Autodesk Inventor part; units mm, degrees
ref_plane "YZ Plane" through (0, 0, 0) normal (1, 0, 0) x (0, 1, 0)
ref_plane "XZ Plane" through (0, 0, 0) normal (0, 1, 0) x (-1, 0, 0)
ref_plane "XY Plane" through (0, 0, 0) normal (0, 0, 1) x (1, 0, 0)
sketch "Sketch1" plane through (0, 0, 0) normal (0, 1, 0) x (-1, 0, 0)
  line L0 (0, 0) -> (-60.96, 0)
  line L1 (-60.96, 0) -> (-60.96, -111.76)
  line L2 (-60.96, -111.76) -> (0, -111.76)
  line L3 (0, -111.76) -> (0, 0)
  dimension "d0" = 60.96
  dimension "d1" = 111.76
extrude "Extrusion1" add sketch "Sketch1" along normal blind 31.75 draft -2
fillet "Fillet1" radius 6.35 4 edges at (60.4056, 15.875, -0.5544) (60.4056, 15.875, -111.2056) (0.5544, 15.875, -111.2056) (0.5544, 15.875, -0.5544)
fillet "Fillet2" radius 0.635 16 edges at (57.993, 31.75, -2.967) (30.48, 31.75, -1.1087) (2.967, 31.75, -2.967) (1.1087, 31.75, -55.88) (2.967, 31.75, -108.793) (30.48, 31.75, -110.6513) (57.993, 31.75, -108.793) (59.8513, 31.75, -55.88) (59.1017, 0, -109.9017) (30.48, 0, -111.76) (1.8583, 0, -109.9017) (0, 0, -55.88) (1.8583, 0, -1.8583) (30.48, 0, 0) (59.1017, 0, -1.8583) (60.96, 0, -55.88)
properties part number "Compressor" material "Aluminum 6061"
Build history of the part. All positions in model axes, mm. Round coordinates to 2 decimals unless told otherwise and drop trailing zeros. Write each loop counter-clockwise with the first axis right and the second up, starting at its lowest first coordinate (ties: lowest second). Pieces come first, ordered by that corner, then holes. Notation, with made-up numbers: (51, 65.25) - (65, 65.25) arc R16 cw to (65, 77.25) - close; hole circle Ø5 at (72.5, -7.5). An arc over 180 degrees is marked (long way). Answer as CSV lines item,"result".
Q1. Drill centre lines: probe 1 along X at (y, z) = (19, -18); probe 2 along Z at (x, y) = (34, 30.5); probe 3 along Z at (x, y) = (39.5, 29.5). Where is each one in solid material? Low to high. Write a range as [from, to].
Report:
probe 1,"x = [0.66, 60.3]"
probe 2,"z = [-110.69, -1.07]"
probe 3,"z = [-110.73, -1.03]"
Q2. Drop flat-ended pins along their axis: pin 1 (10 mm diameter, centred on x = 53, z = -87, fed in from -Y); pin 2 (8 mm diameter, centred on x = 14, y = 27.5, fed in from -Z); pin 3 (6 mm diameter, centred on x = 30.5, y = 14, fed in from +Z); pin 4 (3 mm diameter, centred on x = 17, y = 5.5, fed in from -Z). Give the stop position or say it passes through.
Report:
pin 1,"stops at y = 0"
pin 2,"stops at z = -110.94"
pin 3,"stops at z = -0.38"
pin 4,"stops at z = -111.62"
Q3. Cut at A-A (z = -43.5). Write the cut outline in (x, y) (3 decimals), and give its area (3 significant figures).
Report:
outline,"(0.023, 0.657) arc R0.635 ccw to (0.658, 0) - (60.302, 0) arc R0.635 ccw to (60.937, 0.657) - (59.873, 31.137) arc R0.635 ccw to (59.238, 31.75) - (1.722, 31.75) arc R0.635 ccw to (1.087, 31.137) - close"
area,"1,900 mm^2"
